from build123d import *

# Parameters (mm, degrees)
CROQUIS2_R              = 12.7
SALIENTE_EXTRUIR1_DEPTH = 394.55
CROQUIS4_W              = 45.4
CROQUIS4_H              = 45.4
SALIENTE_EXTRUIR2_DEPTH = 45.4
CROQUIS5_R              = 18.5
CROQUIS5_R_2            = 12.7
SALIENTE_EXTRUIR3_DEPTH = 30
SALIENTE_EXTRUIR4_START = 75.4
CROQUIS7_R              = 18.5
CROQUIS7_R_2            = 12.7
SALIENTE_EXTRUIR4_DEPTH = 75.4


with BuildPart() as part:
    # Croquis2 → Saliente-Extruir1 (new body)
    with BuildSketch(Plane(origin=(0, -12.7, 0), x_dir=(1, 0, 0), z_dir=(0, 1, 0))):
        with Locations(Location((0, -37.25, 0), (0, 0, 270))):
            Circle(CROQUIS2_R)
    extrude(amount=-SALIENTE_EXTRUIR1_DEPTH)

    # Croquis4 → Saliente-Extruir2 (add)
    with BuildSketch(Plane(origin=(0, -12.7, 0), x_dir=(1, 0, 0), z_dir=(0, 1, 0))):
        with Locations((0, -37.25)):
            Rectangle(CROQUIS4_W, CROQUIS4_H)
    extrude(amount=SALIENTE_EXTRUIR2_DEPTH)

    # Croquis5 → Saliente-Extruir3 (add)
    with BuildSketch(Plane(origin=(22.7, 0, 0), x_dir=(0, 0, -1), z_dir=(1, 0, 0))):
        with Locations(Location((-37.25, 10, 0), (0, 0, 180))):
            Circle(CROQUIS5_R)
        with Locations((-37.25, 10)):
            Circle(CROQUIS5_R_2, mode=Mode.SUBTRACT)
    extrude(amount=SALIENTE_EXTRUIR3_DEPTH)

    # Croquis7 → Saliente-Extruir4 (add)
    with BuildSketch(Plane(origin=(0, -12.7, 0), x_dir=(1, 0, 0), z_dir=(0, 1, 0)).offset(SALIENTE_EXTRUIR4_START)):
        with Locations(Location((0, -37.25, 0), (0, 0, 90))):
            Circle(CROQUIS7_R)
        with Locations(Location((0, -37.25, 0), (0, 0, 270))):
            Circle(CROQUIS7_R_2, mode=Mode.SUBTRACT)
    extrude(amount=-SALIENTE_EXTRUIR4_DEPTH)


solid = part.part
CAD build for the part. Positions are in the model's coordinates, mm. A direction names the side the tool comes from. Round coordinates to 2 decimals unless told otherwise and drop trailing zeros. Loops run counter-clockwise (first coordinate to the right, second up) from the corner with the lowest first, then second, coordinate; pieces in that order, holes last.
(1) Cut at A-A (x = 0). Give the cut face in (y, z), plus the area to 3 significant figures.
(2) Two-plate mould, pull along X, no slides. Class faces 5 (the flat face through (22.7, 10, 37)), 6 (the flat face through (0, 32.7, 37)), 7 (the flat face through (0, 10, 14.55)), 8 (the cylindrical face through (3.815, 47.91, 49.364)): +X half, -X half, draft (parallel to the pull), parting line (faces both ways), or undercut.
(3) Wall check: line 1 along Y through (x, z) = (39.5, 37.25); line 2 along Y through (x, z) = (-11, 57); line 3 along Y through (x, z) = (8, 33.5). Give the ranges that are in metal, low to high.
(4) Cut at C-C (z = 37.25). Give the cut face in (x, y), plus the area to 3 significant figures.
(5) Drop flat-ended pins along their axis: pin 1 (8 mm diameter, centred on x = 31.5, z = 35, fed in from -Y); pin 2 (4 mm diameter, centred on y = -163, z = 50.5, fed in from +X); pin 3 (5 mm diameter, centred on x = 13.5, z = 46.5, fed in from -Y). Give the stop position or say it passes through.
(6) Cut at D-D (x = 27.5). Give the cut face in (y, z), plus the area to 3 significant figures.
(7) Which spindle directions (+Z, -Z, +X, -X, +Y, -Y) get a long thin tool onto all of the face, cutting with end or side? Do faces 1 (the cylindrical face through (37.49, -1.267, 31.39)), 2 (the flat face through (52.7, 22.1, 32.9)), 3 (the flat face through (-15.5, 32.7, 26.8)), 4 (the flat face through (-10, -12.7, 47)). Say none if no direction does.
Findings below:
1. outline: (-407.25, 24.55) - (-12.7, 24.55) - (-12.7, 14.55) - (32.7, 14.55) - (32.7, 18.75) - (62.7, 18.75) - (62.7, 24.55) - (32.7, 24.55) - (32.7, 49.95) - (62.7, 49.95) - (62.7, 55.75) - (32.7, 55.75) - (32.7, 59.95) - (-12.7, 59.95) - (-12.7, 49.95) - (-407.25, 49.95) - close
1. area: 12,400 mm2
2. face 5: +X half
2. face 6: undercut
2. face 7: draft
2. face 8: undercut
3. line 1: y = -8.5 to -2.7, 22.7 to 28.5
3. line 2: y = -12.7 to 32.7
3. line 3: y = -407.25 to 32.7
4. outline: (-22.7, -12.7) - (-12.7, -12.7) - (-12.7, -407.25) - (12.7, -407.25) - (12.7, -12.7) - (22.7, -12.7) - (22.7, -8.5) - (52.7, -8.5) - (52.7, -2.7) - (22.7, -2.7) - (22.7, 22.7) - (52.7, 22.7) - (52.7, 28.5) - (22.7, 28.5) - (22.7, 32.7) - (18.5, 32.7) - (18.5, 62.7) - (12.7, 62.7) - (12.7, 32.7) - (-12.7, 32.7) - (-12.7, 62.7) - (-18.5, 62.7) - (-18.5, 32.7) - (-22.7, 32.7) - close
4. area: 12,800 mm2
5. pin 1: stops at y = -8.5
5. pin 2: stops at x = 5.89
5. pin 3: stops at y = -12.7
6. outline: circle Ø37 at (10, 37.25); hole circle Ø25.4 at (10, 37.25)
6. area: 569 mm2
7. face 1: +X
7. face 2: +Z, -Z, +X, +Y, -Y
7. face 3: +Y
7. face 4: -Y
